Verification items for the finished model (mm, model axes). A direction names the side the tool comes from. Coordinates: 2 decimals unless noted, no trailing zeros. Order: outer loops, then holes, each group sorted by start corner. A loop starts at its lowest first (then second) coordinate and runs counter-clockwise, first axis right, second up. Notation, with made-up numbers: M 67.5,54 L 124.5,54 A18 ccw 124.5,58 Z; hole C 43,66 d7. An arc over 180 degrees is marked long. Answer as a JSON object with one key per item and string values. Group by question number.
(1) Cross-section at B-B (y = -1). Enter the section's corners in (x, z), plus the area to 3 significant figures.
(2) Cross-section at A-A (z = 14). Enter the section's corners in (x, y), plus the area to 3 significant figures.
(3) Access from +Z, -Z, +X, -X, +Y, -Y to the whole of each face (thin tool, end or side, straight path). Record for faces 1 (the face through (-6, 6, 8)), 2 (the face through (6, 16, 6)).
(4) Gauge pin test, flat ends, axial feed: pin 1 Ø7 at (x, z) = (-1.5, 17) entering from +Y; pin 2 Ø4 at (y, z) = (4.5, 17) entering from -X; pin 3 Ø6 at (x, y) = (3, 9.5) entering from +Z. Record the tip position at first contact, or that the pin passes through.
(5) Material ranges on line 1 (X direction, y = 10.5, z = 12.25); line 2 (Z direction, x = -16, y = 11.5); line 3 (Y direction, x = 15, z = 13.25), recorded low to high.
from build123d import *

# Parameters (mm, degrees)
ESBO_O1_W                  = 62
ESBO_O1_H                  = 32
ESBO_O1_W_2                = 0.346266541
ESBO_O1_H_2                = 0.178718215
RESSALTO_EXTRUS_O1_DEPTH   = 22
CORTE_EXTRUS_O4_DEPTH      = 42.243181255
CORTE_EXTRUS_O4_DEPTH_BACK = 14
ESBO_O2_W                  = 50
ESBO_O2_H                  = 20


with BuildPart() as part:
    # Esboço1 → Ressalto-extrusão1 (new body)
    with BuildSketch(Plane.XY):
        Rectangle(ESBO_O1_W, ESBO_O1_H)
        with Locations((0.173133271, -0.089359108)):
            Rectangle(ESBO_O1_W_2, ESBO_O1_H_2, mode=Mode.SUBTRACT)
    extrude(amount=RESSALTO_EXTRUS_O1_DEPTH)

    # Esboço2 → Corte-extrusão4 (cut, two sides: drawn at the far end of the back side and taken through both)
    with BuildSketch(Plane.XY.offset(22).offset(-CORTE_EXTRUS_O4_DEPTH_BACK)):
        with Locations((-6, 6)):
            Rectangle(ESBO_O2_W, ESBO_O2_H)
    extrude(amount=CORTE_EXTRUS_O4_DEPTH + CORTE_EXTRUS_O4_DEPTH_BACK, mode=Mode.SUBTRACT)


solid = part.part
Taken from the geometry:
{
 "1": {"outline": "M -31,0 L 31,0 L 31,22 L 19,22 L 19,8 L -31,8 Z", "area": "664 mm²"},
 "2": {"outline": "M -31,-16 L 31,-16 L 31,16 L 19,16 L 19,-4 L -31,-4 Z", "area": "984 mm²"},
 "3": {"face 1": "+Z, -X, +Y", "face 2": "+Z, -Z, +X, -X, +Y"},
 "4": {"pin 1": "stops at y = -4", "pin 2": "stops at x = 19", "pin 3": "stops at z = 8"},
 "5": {"line 1": "x = 19 to 31", "line 2": "z = 0 to 8", "line 3": "y = -16 to -4"}
}
